```python
from build123d import *

# Parameters (mm, degrees)
BOSS_EXTRUDE1_DEPTH   = 7
CUT_EXTRUDE1_REACH    = 36.683
SKETCH2_R             = 2.6
CHAMFER1_SIZE         = 0.5
M4X0_7_TAPPED_HOLE1_D = 3.3


with BuildPart() as part:
    # Sketch1 → Boss-Extrude1 (new, symmetric)
    with BuildSketch(Plane.XY):
        with BuildLine():
            Line((-21, 6.3), (-8.95, 6.3))
            Line((-8.95, 6.3), (-8.95, 33))
            Line((-8.95, 33), (-0.75, 33))
            Line((-0.75, 33), (-0.75, 24.943429983))
            ThreePointArc((-0.75, 24.943429983), (0, 15), (0.75, 24.943429983))
            Line((0.75, 24.943429983), (0.75, 33))
            Line((0.75, 33), (8.95, 33))
            Line((8.95, 33), (8.95, 6.3))
            Line((8.95, 6.3), (21, 6.3))
            Line((21, 6.3), (21, 0))
            Line((21, 0), (-21, 0))
            Line((-21, 0), (-21, 6.3))
        make_face()
    extrude(amount=BOSS_EXTRUDE1_DEPTH, both=True)

    # Sketch2 → Cut-Extrude1 (cut, up to next)
    with BuildSketch(Plane(origin=(0, 6.3, 0), x_dir=(1, 0, 0), z_dir=(0, 1, 0)), mode=Mode.PRIVATE) as cut_extrude1_sk1:
        with Locations(Location((16, 0, 0), (0, 0, 270))):
            Circle(SKETCH2_R)
    cut_extrude1_tool1 = extrude(cut_extrude1_sk1.sketch, amount=-CUT_EXTRUDE1_REACH, mode=Mode.PRIVATE) & part.part
    # Sketch2 → Cut-Extrude1 (cut, up to next)
    with BuildSketch(Plane(origin=(0, 6.3, 0), x_dir=(1, 0, 0), z_dir=(0, 1, 0)), mode=Mode.PRIVATE) as cut_extrude1_sk2:
        with Locations(Location((-16, 0, 0), (0, 0, 270))):
            Circle(SKETCH2_R)
    cut_extrude1_tool2 = extrude(cut_extrude1_sk2.sketch, amount=-CUT_EXTRUDE1_REACH, mode=Mode.PRIVATE) & part.part
    add(cut_extrude1_tool1.solids().sort_by_distance((16, 6.3, 0))[0], mode=Mode.SUBTRACT)
    add(cut_extrude1_tool2.solids().sort_by_distance((-16, 6.3, 0))[0], mode=Mode.SUBTRACT)

    # Chamfer1
    chamfer1_edges = [part.edges().sort_by_distance(p)[0] for p in [
        (16, 6.3, -2.6),
        (-16, 6.3, -2.6),
    ]]
    chamfer(chamfer1_edges, length=CHAMFER1_SIZE)

    # Sketch4 → CBORE for M4 SHCS2 (revolve, cut)
    with BuildSketch(Plane(origin=(8.95, 28, 0), x_dir=(0, 0, -1), z_dir=(0, 1, 0))):
        Polygon((0, 0), (0, 8.2), (2.25, 8.2), (2.25, 4), (4, 4), (4, 0.25), (4.25, 0), align=None)
    revolve(axis=Axis((15.3, 28, 0), (-1, 0, 0)), mode=Mode.SUBTRACT)

    # M4x0.7 Tapped Hole1 (through all)
    with Locations(Plane(origin=(-0.75, 0, 0), x_dir=(0, 0, -1), z_dir=(1, 0, 0))):
        with Locations((0, 28)):
            Hole(M4X0_7_TAPPED_HOLE1_D / 2)


solid = part.part
```
Model file for the job. Use its own axes, mm. A direction names the side the tool comes from. Round coordinates to 2 decimals unless told otherwise and drop trailing zeros. Loops run counter-clockwise (first coordinate to the right, second up) from the corner with the lowest first, then second, coordinate; pieces in that order, holes last. Notation, with made-up numbers: M 56,0.25 L 65,0.25 A12 ccw 65,17.25 Z; hole C 6,76.5 d2. An arc over 180 degrees is marked long. Put each result on its own line as item: value. Start each with the question number.
Item 1: Cut at D-D (z = 0). Give the number of separate pieces and of enclosed holes in the cut face, then the cut area to 3 significant figures.
Item 2: Drop flat-ended pins along their axis: P1, Ø7, axis at y = 24.5, z = -1, coming from the -X side; P2, Ø1, axis at x = 10.5, z = 4, coming from the -Y side; P3, Ø4, axis at y = 28, z = 0, coming from the +X side; P4, Ø4, axis at x = -16, z = 3, coming from the +Y side. Give the stop position or say it passes through.
Item 3: Cut at C-C (x = -5.5). List the corners of the cut face in (y, z).
Item 4: Cut at B-B (y = 28). List the corners of the cut face in (x, z).
Item 5: Drill centre lines: line 1 along Y through (x, z) = (7.4, 0); line 2 along X through (y, z) = (29, -2.5); line 3 along Y through (x, z) = (4.5, -1.25). Where is each one in solid material? Low to high.
Item 6: 3-axis set-ups, long thin cutter, end or side, ignore diameter. For faces 4 (the face through (2.879, 30.196, 0.488)), 5 (the face through (12, 6.3, 0)), 6 (the face through (0.75, 31, 0)), 7 (the face through (-8.95, 19, 0)): which of +Z, -Z, +X, -X, +Y, -Y reach the whole face in a straight line?
Item 7: Cut at A-A (y = 20). List the corners of the cut face in (x, z), then the cut area to 3 significant figures.
Item 8: Mould opens along Z. For faces 1 (the face through (-0.75, 30, 0)), 2 (the face through (4.95, 30, 2)), 3 (the face through (0, 9, 7)) say: released by +Z, released by -Z, zero draft, split by the parting line, or undercut.
Answer block:
1. separate pieces: 5
1. enclosed holes: 0
1. area: 508 mm2
2. P1: x = -8.95
2. P2: y = 0
2. P3: x = -0.75
2. P4: y = 6.3
3. outline: M 0,-7 L 33,-7 L 33,7 L 0,7 Z; hole C 28,0 d3.3
4. outline: M -8.95,-7 L -0.75,-7 L -0.75,-1.65 L -8.95,-1.65 Z; M -8.95,1.65 L -0.75,1.65 L -0.75,7 L -8.95,7 Z; M 0.75,-7 L 8.95,-7 L 8.95,-4.25 L 8.7,-4 L 4.95,-4 L 4.95,-2.25 L 0.75,-2.25 Z; M 0.75,2.25 L 4.95,2.25 L 4.95,4 L 8.7,4 L 8.95,4.25 L 8.95,7 L 0.75,7 Z
5. line 1: 0 to 24, 32 to 33
5. line 2: -8.95 to -0.75, 0.75 to 4.95
5. line 3: 0 to 17.82, 22.18 to 26.13, 29.87 to 33
6. face 4: +X
6. face 5: +Z, -Z, +X, +Y
6. face 6: +Z, -Z, +Y
6. face 7: +Z, -Z, -X, +Y
7. outline: M -8.95,-7 L -5,-7 L -5,7 L -8.95,7 Z; M 5,-7 L 8.95,-7 L 8.95,7 L 5,7 Z
7. area: 111 mm2
8. face 1: zero draft
8. face 2: undercut
8. face 3: released by +Z
